```python
from build123d import *

# Parameters (mm, degrees)
SKETCH1_R           = 3
BOSS_EXTRUDE1_DEPTH = 9
SKETCH3_W           = 8
SKETCH3_H           = 14.926112698
CUT_EXTRUDE1_DEPTH  = 12


with BuildPart() as part:
    # Sketch1 → Boss-Extrude1 (new body)
    with BuildSketch(Plane(origin=(0, 0, 0), x_dir=(0, 0, -1), z_dir=(1, 0, 0))):
        with BuildLine():
            Line((-11.644204214, 4.399749293), (-11.644204214, 14.399749293))
            Line((-11.644204214, 14.399749293), (-1.644204214, 14.399749293))
            Line((-1.644204214, 14.399749293), (-1.644204214, 4.399749293))
            ThreePointArc((-1.644204214, 4.399749293), (-6.644204214, -0.600250707), (-11.644204214, 4.399749293))
        make_face()
        with Locations((-6.644204214, 4.399749293)):
            Circle(SKETCH1_R, mode=Mode.SUBTRACT)
    extrude(amount=BOSS_EXTRUDE1_DEPTH)

    # Sketch3 → Cut-Extrude1 (cut)
    with BuildSketch(Plane(origin=(0, 0, 1.644204214), x_dir=(-1, 0, 0), z_dir=(0, 0, -1))):
        with Locations((-4.5, 5.936692944)):
            Rectangle(SKETCH3_W, SKETCH3_H)
    extrude(amount=-CUT_EXTRUDE1_DEPTH, mode=Mode.SUBTRACT)


solid = part.part
```
Check sheet for the modelled part. Datum: model origin and axes. Units: mm. A direction names the side the tool comes from. Round coordinates to 2 decimals unless told otherwise and drop trailing zeros. Order: outer loops, then holes, each group sorted by start corner. A loop starts at its lowest first (then second) coordinate and runs counter-clockwise, first axis right, second up. Notation, with made-up numbers: M 4,87.25 L 50,87.25 A24 ccw 50,100.25 Z; hole C 52.5,74.25 d5. An arc over 180 degrees is marked long. Answer in a Markdown table with one row per item.
(1) Section check D-D on z = 10.5. Record the boundary of the cut face in (x, y).
Findings:
| item | result |
|---|---|
| outline | M 0,1.22 L 0.5,1.22 L 0.5,13.4 L 8.5,13.4 L 8.5,1.22 L 9,1.22 L 9,14.4 L 0,14.4 Z |
(2) Section check C-C on y = 6. Record the boundary of the cut face in (x, z).
Findings:
| item | result |
|---|---|
| outline | M 0,1.64 L 0.5,1.64 L 0.5,4.11 L 0,4.11 Z; M 0,9.18 L 0.5,9.18 L 0.5,11.64 L 0,11.64 Z; M 8.5,1.64 L 9,1.64 L 9,4.11 L 8.5,4.11 Z; M 8.5,9.18 L 9,9.18 L 9,11.64 L 8.5,11.64 Z |
(3) Material ranges on line 1 along X through (y, z) = (10.5, 11.25); line 2 along Y through (x, z) = (6.5, 7), recorded low to high. Write a range as from..to.
Findings:
| item | result |
|---|---|
| line 1 | x = 0..0.5, 8.5..9 |
| line 2 | y = 13.4..14.4 |
(4) Section check A-A on y = 8.5. Record the boundary of the cut face in (x, z).
Findings:
| item | result |
|---|---|
| outline | M 0,1.64 L 0.5,1.64 L 0.5,11.64 L 0,11.64 Z; M 8.5,1.64 L 9,1.64 L 9,11.64 L 8.5,11.64 Z |
(5) Section check B-B on z = 8. Record the boundary of the cut face in (x, y), plus the area to 3 significant figures.
Findings:
| item | result |
|---|---|
| outline | M 0,-0.41 L 0.5,-0.41 L 0.5,1.72 L 0,1.72 Z; M 0,7.08 L 0.5,7.08 L 0.5,13.4 L 8.5,13.4 L 8.5,7.08 L 9,7.08 L 9,14.4 L 0,14.4 Z; M 8.5,-0.41 L 9,-0.41 L 9,1.72 L 8.5,1.72 Z |
| area | 17.5 mm^2 |
(6) Set-up check for faces 1 (the flat face through (8.5, 8, 7)), 2 (the cylindrical face through (0.2, -0.6, 6.5)): record each of +Z, -Z, +X, -X, +Y, -Y from which the full face is reachable in a straight line by a thin tool's end or side.
Findings:
| item | result |
|---|---|
| face 1 | +Z, -Z, -Y |
| face 2 | +X, -X, -Y |
(7) Draft check along X on faces 3 (the flat face through (4, 14, 1.644)), 4 (the flat face through (9, 9, 7)), 5 (the flat face through (0.5, 8, 7)). Enter one of: +X half, -X half, draft (parallel to the pull), parting line (faces both ways), or undercut.
Findings:
| item | result |
|---|---|
| face 3 | draft |
| face 4 | +X half |
| face 5 | undercut |
(8) Gauge pin test, flat end, axial feed: pin 1 (1 mm diameter, centred on x = 1.5, z = 6, fed in from -Y). Record the tip position at first contact, or that the pin passes through.
Findings:
| item | result |
|---|---|
| pin 1 | stops at y = 13.4 |
